```python
from build123d import *

# Parameters (mm, degrees)
BOSS_EXTRUDE1_DEPTH = 40
SKETCH3_R           = 2.5
CUT_EXTRUDE1_DEPTH  = 6
SKETCH4_R           = 5
CUT_EXTRUDE2_DEPTH  = 6
FILLET1_R           = 1


with BuildPart() as part:
    # Sketch1 → Boss-Extrude1 (new body)
    with BuildSketch(Plane.XY):
        with BuildLine():
            Line((0, 0), (0, 5))
            Line((0, 5), (35, 5))
            Line((35, 5), (35, 40))
            Line((35, 40), (40, 40))
            Line((40, 40), (40, 6.25))
            ThreePointArc((40, 6.25), (38.169417382, 1.830582618), (33.75, 0))
            Line((33.75, 0), (0, 0))
        make_face()
    extrude(amount=BOSS_EXTRUDE1_DEPTH)

    # Sketch3 → Cut-Extrude1 (cut, through all)
    with BuildSketch(Plane(origin=(0, 5, 0), x_dir=(1, 0, 0), z_dir=(0, 1, 0))):
        with Locations((15, -10)):
            Circle(SKETCH3_R)
        with Locations((15, -30)):
            Circle(SKETCH3_R)
    extrude(amount=-CUT_EXTRUDE1_DEPTH, mode=Mode.SUBTRACT)

    # Sketch4 → Cut-Extrude2 (cut, through all)
    with BuildSketch(Plane.ZY.offset(-35)):
        with Locations((20, 25)):
            Circle(SKETCH4_R)
    extrude(amount=-CUT_EXTRUDE2_DEPTH, mode=Mode.SUBTRACT)

    # Fillet1
    fillet1_edges = [part.edges().sort_by_distance(p)[0] for p in [
        (35, 5, 20),
    ]]
    fillet(fillet1_edges, radius=FILLET1_R)


solid = part.part
```
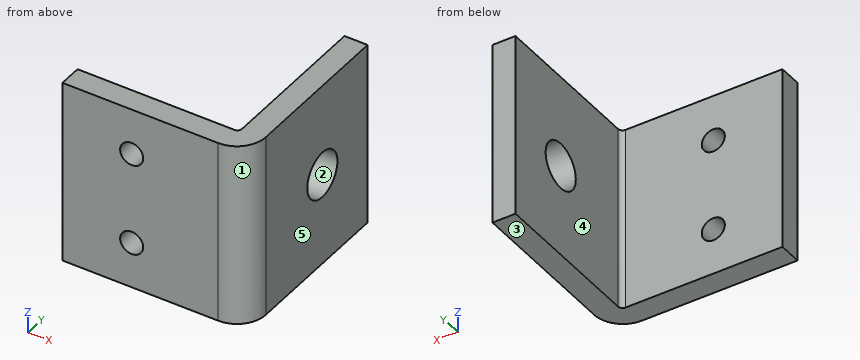
Geometry: final body of the model. Coordinates: model frame, mm. Face numbers are marked on the shaded views. A direction names the side the tool comes from. Give positions to 0.01 mm unless a question says otherwise; leave off trailing zeros. Order: outer loops, then holes, each group sorted by start corner. A loop starts at its lowest first (then second) coordinate and runs counter-clockwise, first axis right, second up. Notation, with made-up numbers: M 69.5,-31.75 L 97.5,-31.75 A34 ccw 97.5,6.25 Z; hole C 19,1 d6. An arc over 180 degrees is marked long. Answer as CSV lines item,"result". Start each with the question number.
1) Cut plane D-D (z = 20). Output: boundary loops of the cut face in (x, y), then the cut area to 3 significant figures.
2) Cut plane A-A (z = 10). Output: boundary loops of the cut face in (x, y), then the cut area to 3 significant figures.
3) Cut plane C-C (y = 25). Output: boundary loops of the cut face in (x, z), then the cut area to 3 significant figures.
4) First-contact query: P1, Ø6, axis at x = 11.5, y = 9.5, coming from the -Z side; P2, Ø10, axis at x = 34.5, z = 31, coming from the -Y side; P3, Ø6.5, axis at x = 15, z = 10, coming from the +Y side; P4, Ø17, axis at y = 29, z = 15, coming from the -X side. Flat tips, straight axial feed; report the tip coordinate or a pass-through.
5) Cut plane B-B (x = 15). Output: boundary loops of the cut face in (y, z).
6) Set-up query: the marked faces 4 and 5. Return all of +Z, -Z, +X, -X, +Y, -Y with unobstructed straight access to the full face (end or side cutting, diameter ignored); none if empty.
7) Line query: line 1 (Z direction, x = 15, y = 2.9); line 2 (X direction, y = 10, z = 25.5); line 3 (Y direction, x = 22.5, z = 14). Output: solid intervals per line, ascending. Write a range as from..to.
8) Mould query, pull axis Y, two halves, no side actions, for the marked faces 1, 2 and 3. Classes: +Y half, -Y half, draft (parallel to the pull), parting line (faces both ways), or undercut.
Findings below:
1,outline,"M 0,0 L 33.75,0 A6.25 ccw 40,6.25 L 40,20 L 35,20 L 35,6 A1 cw 34,5 L 0,5 Z; M 35,30 L 40,30 L 40,40 L 35,40 Z"
1,area,"317 mm²"
2,outline,"M 0,0 L 12.5,0 L 12.5,5 L 0,5 Z; M 17.5,0 L 33.75,0 A6.25 ccw 40,6.25 L 40,40 L 35,40 L 35,6 A1 cw 34,5 L 17.5,5 Z"
2,area,"342 mm²"
3,outline,"M 35,0 L 40,0 L 40,15 L 35,15 Z; M 35,25 L 40,25 L 40,40 L 35,40 Z"
3,area,"150 mm²"
4,P1,"passes through"
4,P2,"stops at y = 0"
4,P3,"stops at y = 5"
4,P4,"stops at x = 35"
5,outline,"M 0,0 L 5,0 L 5,7.5 L 0,7.5 Z; M 0,12.5 L 5,12.5 L 5,27.5 L 0,27.5 Z; M 0,32.5 L 5,32.5 L 5,40 L 0,40 Z"
6,face 4,"+Z, -Z, -X, +Y"
6,face 5,"+Z, -Z, +X, +Y, -Y"
7,line 1,"z = 0..7.5, 12.5..27.5, 32.5..40"
7,line 2,"x = 35..40"
7,line 3,"y = 0..5"
8,face 1,"-Y half"
8,face 2,"undercut"
8,face 3,"draft"
